```python
from build123d import *

# Parameters (mm, degrees)
SKETCH_1_W               = 30
SKETCH_1_H               = 30
EXTRUDE_1_DEPTH          = 140
SKETCH_2_W               = 28
SKETCH_2_H               = 28
CUT_EXTRUDE_1_DEPTH      = 141
CUT_EXTRUDE_1_DEPTH_BACK = 141
SKETCH_3_R               = 2.025
CUT_EXTRUDE_2_DEPTH      = 1
CUT_EXTRUDE_2_DEPTH_BACK = 31
SKETCH_5_R               = 2.025
CUT_EXTRUDE_3_DEPTH      = 31
SKETCH_6_R               = 2.025
CUT_EXTRUDE_4_DEPTH      = 1
SKETCH_7_W               = 18
SKETCH_7_H               = 18
CUT_EXTRUDE_5_DEPTH      = 1
FILLET_1_R               = 2
SKETCH_8_R               = 2.025
CUT_EXTRUDE_6_DEPTH      = 10
SKETCH_10_R              = 7.5
SKETCH_10_R_2            = 6.5
CUT_EXTRUDE_7_DEPTH      = 1
CUT_EXTRUDE_7_DEPTH_BACK = 31
CUT_EXTRUDE_8_DEPTH      = 1
CUT_EXTRUDE_8_DEPTH_BACK = 31
CUT_EXTRUDE_START        = 29
SKETCH_12_R              = 2.025
CUT_EXTRUDE_9_DEPTH      = 10


with BuildPart() as part:
    # 草图1 → 凸台-拉伸1 (new body, symmetric)
    with BuildSketch(Plane(origin=(0, 0, 0), x_dir=(1, 0, 0), z_dir=(0, 1, 0))):
        Rectangle(SKETCH_1_W, SKETCH_1_H)
    extrude(amount=EXTRUDE_1_DEPTH, both=True)

    # 草图2 → 切除-拉伸1 (cut, two sides)
    with BuildSketch(Plane(origin=(0, 0, 0), x_dir=(1, 0, 0), z_dir=(0, 1, 0))) as cut_extrude_1_sk:
        Rectangle(SKETCH_2_W, SKETCH_2_H)
    extrude(amount=CUT_EXTRUDE_1_DEPTH, mode=Mode.SUBTRACT)
    extrude(cut_extrude_1_sk.sketch, amount=-CUT_EXTRUDE_1_DEPTH_BACK, mode=Mode.SUBTRACT)

    # 草图3 → 切除-拉伸2 (cut, two sides)
    with BuildSketch(Plane.ZY.offset(15)) as cut_extrude_2_sk:
        with Locations((0, -78.5)):
            Circle(SKETCH_3_R)
        with Locations((0, -109.5)):
            Circle(SKETCH_3_R)
        with Locations((0, -136)):
            Circle(SKETCH_3_R)
    extrude(amount=CUT_EXTRUDE_2_DEPTH, mode=Mode.SUBTRACT)
    extrude(cut_extrude_2_sk.sketch, amount=-CUT_EXTRUDE_2_DEPTH_BACK, mode=Mode.SUBTRACT)

    # 草图5 → 切除-拉伸3 (cut, through all)
    with BuildSketch(Plane.ZY.offset(15)):
        with Locations((0, 136)):
            Circle(SKETCH_5_R)
        with Locations((0, 111)):
            Circle(SKETCH_5_R)
        with Locations((0, 84)):
            Circle(SKETCH_5_R)
    extrude(amount=-CUT_EXTRUDE_3_DEPTH, mode=Mode.SUBTRACT)

    # 草图6 → 切除-拉伸4 (cut)
    with BuildSketch(Plane(origin=(0, 0, -15), x_dir=(-1, 0, 0), z_dir=(0, 0, -1))):
        with Locations((0, 95)):
            Circle(SKETCH_6_R)
        with Locations((0, 125)):
            Circle(SKETCH_6_R)
    extrude(amount=-CUT_EXTRUDE_4_DEPTH, mode=Mode.SUBTRACT)

    # 草图7 → 切除-拉伸5 (cut)
    with BuildSketch(Plane(origin=(0, 0, 14), x_dir=(-1, 0, 0), z_dir=(0, 0, -1))):
        with Locations((0, 95)):
            Rectangle(SKETCH_7_W, SKETCH_7_H)
    extrude(amount=-CUT_EXTRUDE_5_DEPTH, mode=Mode.SUBTRACT)

    # 圆角1
    fillet_1_edges = [part.edges().sort_by_distance(p)[0] for p in [
        (-9, 104, 14.5),
        (-9, 86, 14.5),
        (9, 86, 14.5),
        (9, 104, 14.5),
    ]]
    fillet(fillet_1_edges, radius=FILLET_1_R)

    # 草图8 → 切除-拉伸6 (cut)
    with BuildSketch(Plane(origin=(0, 0, -15), x_dir=(-1, 0, 0), z_dir=(0, 0, -1))):
        with Locations((0, 136)):
            Circle(SKETCH_8_R)
    extrude(amount=-CUT_EXTRUDE_6_DEPTH, mode=Mode.SUBTRACT)

    # 草图10 → 切除-拉伸7 (cut, two sides)
    with BuildSketch(Plane.ZY.offset(15)) as cut_extrude_7_sk:
        with Locations((0, 96)):
            Circle(SKETCH_10_R)
        with Locations((0, 125)):
            Circle(SKETCH_10_R_2)
    extrude(amount=CUT_EXTRUDE_7_DEPTH, mode=Mode.SUBTRACT)
    extrude(cut_extrude_7_sk.sketch, amount=-CUT_EXTRUDE_7_DEPTH_BACK, mode=Mode.SUBTRACT)

    # 草图11 → 切除-拉伸8 (cut, two sides)
    with BuildSketch(Plane(origin=(0, 0, -15), x_dir=(-1, 0, 0), z_dir=(0, 0, -1))) as cut_extrude_8_sk:
        with BuildLine():
            Line((-8, -115), (-8, -95))
            ThreePointArc((-8, -95), (0, -87), (8, -95))
            Line((8, -95), (8, -115))
            ThreePointArc((8, -115), (0, -123), (-8, -115))
        make_face()
    extrude(amount=CUT_EXTRUDE_8_DEPTH, mode=Mode.SUBTRACT)
    extrude(cut_extrude_8_sk.sketch, amount=-CUT_EXTRUDE_8_DEPTH_BACK, mode=Mode.SUBTRACT)

    # 草图12 → 切除-拉伸9 (cut)
    with BuildSketch(Plane.XY.offset(-14).offset(CUT_EXTRUDE_START)):
        with Locations((-7.5, 136)):
            Circle(SKETCH_12_R)
        with Locations((7.5, 136)):
            Circle(SKETCH_12_R)
    extrude(amount=-CUT_EXTRUDE_9_DEPTH, mode=Mode.SUBTRACT)


solid = part.part
```
The model under review builds one solid part; all positions refer to its coordinate system, in mm. A direction names the side the tool comes from. Round coordinates to 2 decimals unless told otherwise and drop trailing zeros. Write each loop counter-clockwise with the first axis right and the second up, starting at its lowest first coordinate (ties: lowest second). Pieces come first, ordered by that corner, then holes. Notation, with made-up numbers: M -40,89 L -12,89 A11 cw -12,100 Z; hole C 21.5,25.25 d9. An arc over 180 degrees is marked long. Use CSV: the item, a comma, the result in double quotes. Start each with the question number.
(1) The part is to be moulded in two halves that separate along X. For faces 4 (the face through (-15, 2, 0)), 5 (the face through (-0.176, -122.998, -14.507)), 6 (the face through (0.176, -87.002, -14.507)), 7 (the face through (-14.507, 129.393, -4.791)), say which applies: +X half, -X half, draft (parallel to the pull), parting line (faces both ways), or undercut.
(2) For line 1 along Z through (x, y) = (12.5, -50); line 2 along Z through (x, y) = (14.6, -136) (3 decimals), list the stretches that pass through material, from the lowest coordinate up.
(3) We need section A-A, the plane y = -52. State the section outline as (x, z) points, then the cut area to 3 significant figures.
(4) Tool access review of faces 1 (the face through (-14, 2, 0)), 2 (the face through (14.49, 88.68, -1.63)), 3 (the face through (0.176, -87.002, 14.493)): name each direction out of +Z, -Z, +X, -X, +Y, -Y from which nothing blocks a thin tool from reaching the whole face with its end or side.
(5) Clearance check with flat-ended pins moving along their axes: P1, Ø5, axis at x = -0.5, z = 10, coming from the +Y side; P2, Ø3, axis at x = 0, y = 125, coming from the -Z side. State where each tip first meets the part, or that it passes through.
Findings:
1,face 4,"-X half"
1,face 5,"undercut"
1,face 6,"undercut"
1,face 7,"draft"
2,line 1,"-15 to -14, 14 to 15"
2,line 2,"-15 to -2.025, 2.025 to 15"
3,outline,"M -15,-15 L 15,-15 L 15,15 L -15,15 Z; hole M -14,-14 L 14,-14 L 14,14 L -14,14 Z"
3,area,"116 mm^2"
4,face 1,"+Y, -Y"
4,face 2,"+X, -X"
4,face 3,"+Z, -Z"
5,P1,"through"
5,P2,"z = 14"
